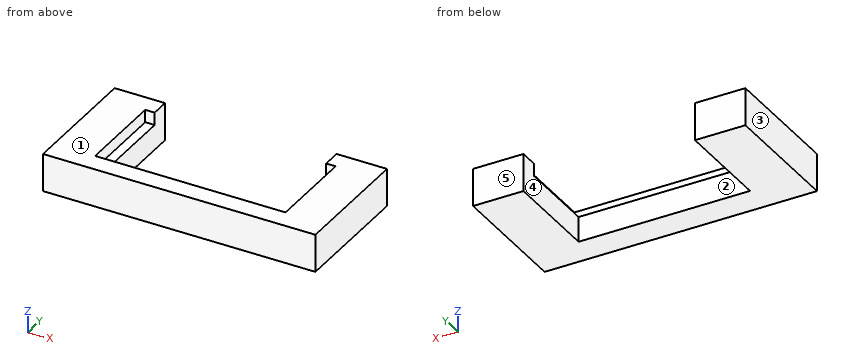
from build123d import *

# Parameters (mm, degrees)
F1_DEPTH = 3
F3_DEPTH = 1


with BuildPart() as f1:
    # F0 (on Top) → F1 (new body)
    with BuildSketch(Plane.XY):
        Polygon((0, 10), (0, 0), (21.6, 0), (21.6, 10), (17.6, 10), (17.6, 2.3), (4, 2.3), (4, 10), align=None)
    extrude(amount=F1_DEPTH)

    # F2 (on face) → F3 (cut)
    with BuildSketch(Plane.XY.offset(3)):
        Polygon((4, 2.3), (4, 8.55), (3.25, 8.55), (3.25, 1.55), (18.35, 1.55), (18.35, 8.55), (17.6, 8.55), (17.6, 2.3), align=None)
    extrude(amount=-F3_DEPTH, mode=Mode.SUBTRACT)


solid = f1.part
Check sheet for the modelled part. Datum: model origin and axes. Units: mm. Face numbers are marked on the shaded views. A direction names the side the tool comes from. Round coordinates to 2 decimals unless told otherwise and drop trailing zeros. Loops run counter-clockwise (first coordinate to the right, second up) from the corner with the lowest first, then second, coordinate; pieces in that order, holes last.
1. Mould release check, pull along X, two halves, no side actions. Record for the marked faces 1, 2 and 3: released by +X, released by -X, zero draft, split by the parting line, or undercut.
2. Sectioned sample at D-D on z = 1.3. Record the boundary of the cut face in (x, y), and give its area (3 significant figures).
3. Sectioned sample at B-B on z = 2.35. Record the boundary of the cut face in (x, y).
4. Sectioned sample at A-A on y = 8.25. Record the boundary of the cut face in (x, z).
5. Scan lines: probe 1 along X at (y, z) = (6.75, 2.05); probe 2 along X at (y, z) = (6, 1.7); probe 3 along Y at (x, z) = (18, 2.2). Record each from-to range of solid material in increasing order.
6. Set-up check for the marked faces 4 and 5: record each of +Z, -Z, +X, -X, +Y, -Y from which the full face is reachable in a straight line by a thin tool's end or side.
7. Gauge pin test, flat end, axial feed: pin 1 Ø0.6 at (x, z) = (10, 0.5) entering from +Y. Record the tip position at first contact, or that the pin passes through.
8. Sectioned sample at C-C on x = 3.5. Record the boundary of the cut face in (y, z), and give its area (3 significant figures).
Recorded:
1. face 1: zero draft
1. face 2: undercut
1. face 3: released by -X
2. outline: (0, 0) - (21.6, 0) - (21.6, 10) - (17.6, 10) - (17.6, 2.3) - (4, 2.3) - (4, 10) - (0, 10) - close
2. area: 111 mm2
3. outline: (0, 0) - (21.6, 0) - (21.6, 10) - (17.6, 10) - (17.6, 8.55) - (18.35, 8.55) - (18.35, 1.55) - (3.25, 1.55) - (3.25, 8.55) - (4, 8.55) - (4, 10) - (0, 10) - close
4. outline: (0, 0) - (4, 0) - (4, 2) - (3.25, 2) - (3.25, 3) - (0, 3) - close; (17.6, 0) - (21.6, 0) - (21.6, 3) - (18.35, 3) - (18.35, 2) - (17.6, 2) - close
5. probe 1: x = 0 to 3.25, 18.35 to 21.6
5. probe 2: x = 0 to 4, 17.6 to 21.6
5. probe 3: y = 0 to 1.55, 8.55 to 10
6. face 4: +Z, -Z, +Y
6. face 5: +Z, -Z, +X, -X, +Y
7. pin 1: stops at y = 2.3
8. outline: (0, 0) - (10, 0) - (10, 3) - (8.55, 3) - (8.55, 2) - (1.55, 2) - (1.55, 3) - (0, 3) - close
8. area: 23.0 mm2
